Build history of the part. All positions in model axes, mm. Face numbers are marked on the shaded views. A direction names the side the tool comes from. Give positions to 0.01 mm unless a question says otherwise; leave off trailing zeros. Loops run counter-clockwise (first coordinate to the right, second up) from the corner with the lowest first, then second, coordinate; pieces in that order, holes last. Notation, with made-up numbers: (4.5, 19) -> (13.5, 19) arc R20 cw to (13.5, 35) -> close; hole circle Ø1 at (32, 3). An arc over 180 degrees is marked (long way). Answer as a JSON object with one key per item and string values. Group by question number.
from build123d import *

# Parameters (mm, degrees)
SKETCH_W        = 23
SKETCH_H        = 23
PAD_DEPTH       = 23
SKETCH001_W     = 21
SKETCH001_H     = 21
POCKET_DEPTH    = 18.6
SKETCH002_R     = 1.7
POCKET001_DEPTH = 5
SKETCH003_W     = 23
SKETCH003_H     = 1.8
PAD001_DEPTH    = 5
SKETCH004_W     = 23
SKETCH004_H     = 1.8
PAD002_DEPTH    = 5
FILLET_R        = 5


with BuildPart() as part:
    # Sketch → Pad (new body)
    with BuildSketch(Plane.XY):
        Rectangle(SKETCH_W, SKETCH_H)
    extrude(amount=PAD_DEPTH)

    # Sketch001 (on Face6 of Pad) → Pocket (cut)
    with BuildSketch(Plane.XY.offset(23)):
        Rectangle(SKETCH001_W, SKETCH001_H)
    extrude(amount=-POCKET_DEPTH, mode=Mode.SUBTRACT)

    # Sketch002 (on Face4 of Pocket) → Pocket001 (cut)
    with BuildSketch(Plane(origin=(0, 0, 0), x_dir=(1, 0, 0), z_dir=(0, 0, -1))):
        Circle(SKETCH002_R)
        with Locations((7.62, 0)):
            Circle(SKETCH002_R)
        with Locations((-7.62, 0)):
            Circle(SKETCH002_R)
    extrude(amount=-POCKET001_DEPTH, mode=Mode.SUBTRACT)

    # Sketch003 (on Face1 of Pocket001) → Pad001 (join)
    with BuildSketch(Plane(origin=(-11.5, 0, 0), x_dir=(0, -1, 0), z_dir=(-1, 0, 0))):
        with Locations((0, 10.9)):
            Rectangle(SKETCH003_W, SKETCH003_H)
    extrude(amount=PAD001_DEPTH)

    # Sketch004 (on Face6 of Pad001) → Pad002 (join)
    with BuildSketch(Plane.YZ.offset(11.5)):
        with Locations((0, 10.9)):
            Rectangle(SKETCH004_W, SKETCH004_H)
    extrude(amount=PAD002_DEPTH)

    # Fillet
    fillet_edges = [part.edges().sort_by_distance(p)[0] for p in [
        (16.5, -11.5, 10.9),
        (16.5, 11.5, 10.9),
        (-16.5, -11.5, 10.9),
        (-16.5, 11.5, 10.9),
    ]]
    fillet(fillet_edges, radius=FILLET_R)


solid = part.part
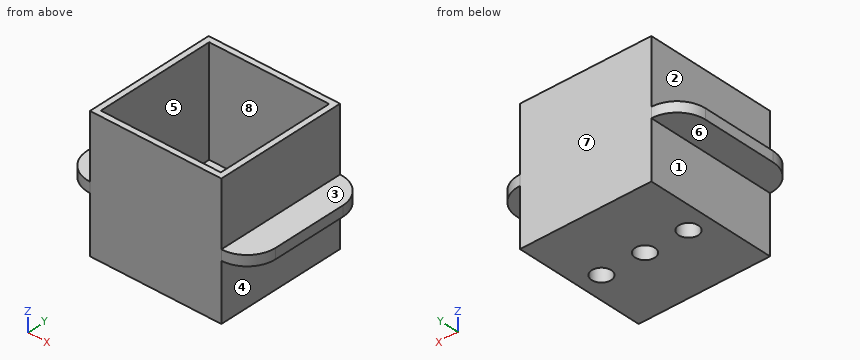
(1) 3-axis set-ups, long thin cutter, end or side, ignore diameter. For the marked faces 1, 2, 3 and 4: which of +Z, -Z, +X, -X, +Y, -Y reach the whole face in a straight line?
(2) Saw through at C-C on y = 0. List the corners of the cut face in (x, z).
(3) Pin check, flat tips, straight feed: pin 1 (8 mm diameter, centred on y = 0, z = 2.5, fed in from -X); pin 2 (2 mm diameter, centred on x = 7.62, y = 0, fed in from +Z); pin 3 (4 mm diameter, centred on x = 15, y = -2, fed in from -Z); pin 4 (1.5 mm diameter, centred on x = 15, y = -3, fed in from +Z). Stop position of each tip, or through.
(4) Pull direction Y, two halves, no side cores. Call the marked faces 5, 6, 7 and 8: pulls with the +Y half, pulls with the -Y half, needs draft (parallel to the pull), parting line crosses it, or undercut.
(5) Probe line 1 along X through (y, z) = (0, 2.05); line 2 along Y through (x, z) = (0, 14). List the from-to ranges inside material, lowest first. Write a range as [from, to].
(6) Saw through at B-B on x = 0. List the corners of the cut face in (y, z), plus the area to 3 significant figures.
(7) Saw through at A-A on z = 16.25. List the corners of the cut face in (x, y).
(8) Saw through at D-D on y = 3.5. List the corners of the cut face in (x, z).
Calculated:
{
 "1": {"face 1": "-Z, -X, +Y, -Y", "face 2": "+Z, -X, +Y, -Y", "face 3": "+Z, +X, +Y, -Y", "face 4": "-Z, +X, +Y, -Y"},
 "2": {"outline": "(-16.5, 10) -> (-11.5, 10) -> (-11.5, 0) -> (-9.32, 0) -> (-9.32, 4.4) -> (-10.5, 4.4) -> (-10.5, 23) -> (-11.5, 23) -> (-11.5, 11.8) -> (-16.5, 11.8) -> close; (-5.92, 0) -> (-1.7, 0) -> (-1.7, 4.4) -> (-5.92, 4.4) -> close; (1.7, 0) -> (5.92, 0) -> (5.92, 4.4) -> (1.7, 4.4) -> close; (9.32, 0) -> (11.5, 0) -> (11.5, 10) -> (16.5, 10) -> (16.5, 11.8) -> (11.5, 11.8) -> (11.5, 23) -> (10.5, 23) -> (10.5, 4.4) -> (9.32, 4.4) -> close"},
 "3": {"pin 1": "stops at x = -11.5", "pin 2": "passes through", "pin 3": "stops at z = 10", "pin 4": "stops at z = 11.8"},
 "4": {"face 5": "undercut", "face 6": "needs draft", "face 7": "pulls with the +Y half", "face 8": "undercut"},
 "5": {"line 1": "x = [-11.5, -9.32], [-5.92, -1.7], [1.7, 5.92], [9.32, 11.5]", "line 2": "y = [-11.5, -10.5], [10.5, 11.5]"},
 "6": {"outline": "(-11.5, 0) -> (-1.7, 0) -> (-1.7, 4.4) -> (-10.5, 4.4) -> (-10.5, 23) -> (-11.5, 23) -> close; (1.7, 0) -> (11.5, 0) -> (11.5, 23) -> (10.5, 23) -> (10.5, 4.4) -> (1.7, 4.4) -> close", "area": "123 mm^2"},
 "7": {"outline": "(-11.5, -11.5) -> (11.5, -11.5) -> (11.5, 11.5) -> (-11.5, 11.5) -> close; hole (-10.5, -10.5) -> (10.5, -10.5) -> (10.5, 10.5) -> (-10.5, 10.5) -> close"},
 "8": {"outline": "(-16.5, 10) -> (-11.5, 10) -> (-11.5, 0) -> (11.5, 0) -> (11.5, 10) -> (16.5, 10) -> (16.5, 11.8) -> (11.5, 11.8) -> (11.5, 23) -> (10.5, 23) -> (10.5, 4.4) -> (-10.5, 4.4) -> (-10.5, 23) -> (-11.5, 23) -> (-11.5, 11.8) -> (-16.5, 11.8) -> close"}
}
